Geometry check sheet. Reference: the model listing, model coordinates, mm. Face numbers are marked on the shaded views. A direction names the side the tool comes from. Give positions to 0.01 mm unless a question says otherwise; leave off trailing zeros. Loops run counter-clockwise (first coordinate to the right, second up) from the corner with the lowest first, then second, coordinate; pieces in that order, holes last. Notation, with made-up numbers: (14.25, -5.5) -> (24.25, -5.5) arc R25 cw to (24.25, 28.5) -> close; hole circle Ø5 at (41, 56). An arc over 180 degrees is marked (long way). Answer as a JSON object with one key per item and string values.
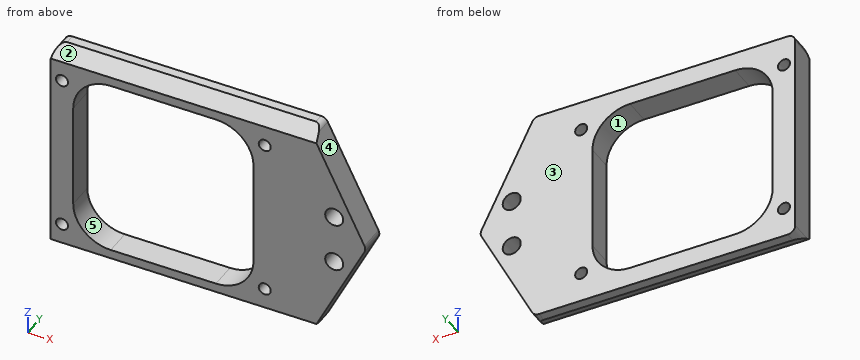
from build123d import *

# Parameters (mm, degrees)
BOSS_EXTRUDE1_DEPTH     = 1.75
CUT_EXTRUDE1_DEPTH      = 52.069193258
CUT_EXTRUDE1_DEPTH_BACK = 52.069193258
SKETCH2_W               = 24
SKETCH2_H               = 24
FILLET1_R               = 5
M2X0_4_TAPPED_HOLE1_D   = 1.6
FILLET2_R               = 1
SKETCH11_W              = 39.153964454
SKETCH11_H              = 3.647114317
CUT_EXTRUDE2_DEPTH      = 51.858555782
M2_CLEARANCE_HOLE2_D    = 2.4


with BuildPart() as part:
    # Sketch1 → Boss-Extrude1 (new, symmetric)
    with BuildSketch(Plane(origin=(0, 0, 0), x_dir=(1, 0, 0), z_dir=(0, 1, 0))):
        Polygon((0, 0), (34.748434417, 0), (42, 14.5), (34.748434417, 29), (0, 29), align=None)
    extrude(amount=BOSS_EXTRUDE1_DEPTH, both=True)

    # Sketch2 → Cut-Extrude1 (cut, two sides: drawn at the far end of the back side and taken through both)
    with BuildSketch(Plane(origin=(0, 0, 0), x_dir=(1, 0, 0), z_dir=(0, 1, 0)).offset(-CUT_EXTRUDE1_DEPTH_BACK)):
        with Locations((15, 14.5)):
            Rectangle(SKETCH2_W, SKETCH2_H)
    extrude(amount=CUT_EXTRUDE1_DEPTH + CUT_EXTRUDE1_DEPTH_BACK, mode=Mode.SUBTRACT)

    # Fillet1
    fillet1_edges = [part.edges().sort_by_distance(p)[0] for p in [
        (3, 0, -2.5),
        (3, 0, -26.5),
        (27, 0, -26.5),
        (27, 0, -2.5),
    ]]
    fillet(fillet1_edges, radius=FILLET1_R)

    # M2x0.4 Tapped Hole1 (through all)
    with Locations(Plane(origin=(1.5, 1.75, -25), x_dir=(0, 0, 1), z_dir=(0, 1, 0))):
        with Locations((0, 0), (0, 27), (7.25, 36.248434417), (13.75, 36.248434417), (21, 27), (21, 0)):
            Hole(M2X0_4_TAPPED_HOLE1_D / 2)

    # Fillet2
    fillet2_edges = [part.edges().sort_by_distance(p)[0] for p in [
        (0, 0, -29),
        (34.748434417, 0, -29),
        (42, 0, -14.5),
        (34.748434417, 0, 0),
        (0, 0, 0),
    ]]
    fillet(fillet2_edges, radius=FILLET2_R)

    # Sketch11 → Cut-Extrude2 (cut, through all)
    with BuildSketch(Plane(origin=(0, 0.119868355, -0.207618081), x_dir=(1, 0, 0), z_dir=(9.104401052367775e-15, -0.5000000000000047, 0.866025403784436))):
        with Locations((19.576982227, -0.335580838)):
            Rectangle(SKETCH11_W, SKETCH11_H)
    cut_extrude2 = extrude(amount=CUT_EXTRUDE2_DEPTH, mode=Mode.SUBTRACT)

    # Mirror1: Cut-Extrude2 across plane
    add(cut_extrude2.mirror(Plane(origin=(0, 0, -14.5), x_dir=(1, 0, 0), z_dir=(0, 0, -1))), mode=Mode.SUBTRACT)

    # M2 Clearance Hole2 (through all)
    with Locations(Plane(origin=(37.748434417, 1.75, -17.75), x_dir=(0, 0, 1), z_dir=(0, 1, 0))):
        with Locations((0, 0), (6.5, 0)):
            Hole(M2_CLEARANCE_HOLE2_D / 2)


solid = part.part
1) Section check A-A on x = 28.5. Record the cut outline in (y, z).
Geometry check:
{"outline": "(-1.75, -27.71) -> (0.48, -29) -> (1.75, -29) -> (1.75, -25.8) -> (-1.75, -25.8) -> close; (-1.75, -24.2) -> (1.75, -24.2) -> (1.75, -4.8) -> (-1.75, -4.8) -> close; (-1.75, -3.2) -> (1.75, -3.2) -> (1.75, 0) -> (0.48, 0) -> (-1.75, -1.29) -> close"}
2) Material ranges on line 1 along X through (y, z) = (-0.85, -14.5); line 2 along X through (y, z) = (0.9, -25); line 3 along X through (y, z) = (-0.1, -17.75), recorded low to high. Write a range as from..to.
Geometry check:
{"line 1": "x = 0..3, 27..41.88", "line 2": "x = 0..0.7, 2.3..4.43, 25.57..27.7, 29.3..36.75", "line 3": "x = 0..3, 27..36.55, 38.95..40.37"}
3) Section check C-C on z = -25. Record the cut outline in (x, y).
Geometry check:
{"outline": "(0, -1.75) -> (0.7, -1.75) -> (0.7, 1.75) -> (0, 1.75) -> close; (2.3, -1.75) -> (4.43, -1.75) -> (4.43, 1.75) -> (2.3, 1.75) -> close; (25.57, -1.75) -> (27.7, -1.75) -> (27.7, 1.75) -> (25.57, 1.75) -> close; (29.3, -1.75) -> (36.75, -1.75) -> (36.75, 1.75) -> (29.3, 1.75) -> close"}
4) Section check B-B on z = -8. Record the cut outline in (x, y).
Geometry check:
{"outline": "(0, -1.75) -> (3, -1.75) -> (3, 1.75) -> (0, 1.75) -> close; (27, -1.75) -> (38.75, -1.75) -> (38.75, 1.75) -> (27, 1.75) -> close"}
5) Depth check by flat-ended pin: P1, Ø1, axis at y = -0.5, z = -8, coming from the +X side; P2, Ø1.8, axis at y = 0.5, z = -16, coming from the +X side; P3, Ø1, axis at x = 14, y = -0.5, coming from the +Z side. Enter the tip coordinate at first touch or a pass-through.
Geometry check:
{"P1": "stops at x = 39", "P2": "stops at x = 41.7", "P3": "stops at z = -0.28"}
6) Draft check along X on the marked faces 3, 4 and 5. Enter one of: pulls with the +X half, pulls with the -X half, needs draft (parallel to the pull), parting line crosses it, or undercut.
Geometry check:
{"face 3": "needs draft", "face 4": "pulls with the +X half", "face 5": "undercut"}
7) Tool access check on the marked faces 1 and 2. Record the directions out of +Z, -Z, +X, -X, +Y, -Y that give a thin tool (end or side, any length) a straight path to the whole face; none if there is none.
Geometry check:
{"face 1": "+Y, -Y", "face 2": "+Z, +X, -X, -Y"}
8) Section check D-D on x = 13. Record the cut outline in (y, z), plus the area to 3 significant figures.
Geometry check:
{"outline": "(-1.75, -27.71) -> (0.48, -29) -> (1.75, -29) -> (1.75, -26.5) -> (-1.75, -26.5) -> close; (-1.75, -2.5) -> (1.75, -2.5) -> (1.75, 0) -> (0.48, 0) -> (-1.75, -1.29) -> close", "area": "14.6 mm2"}
